Verification items for the finished model (mm, model axes). Round coordinates to 2 decimals unless told otherwise and drop trailing zeros. Write each loop counter-clockwise with the first axis right and the second up, starting at its lowest first coordinate (ties: lowest second). Pieces come first, ordered by that corner, then holes.
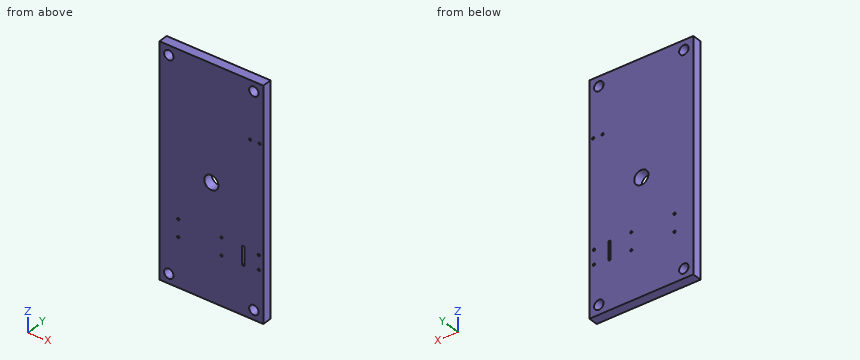
from build123d import *

# Parameters (mm, degrees)
SKETCH1_W                      = 139.7
SKETCH1_H                      = 304.8
BOSS_EXTRUDE1_DEPTH            = 12.7
SKETCH5_R                      = 6.35
CUT_EXTRUDE2_DEPTH             = 13.7
F_3_4_0_7500_DOWEL_HOLE1_D     = 19.05
F_3_4_0_7500_DOWEL_HOLE1_DEPTH = 25.4
F_3_4_0_7500_DOWEL_HOLE1_TIP   = 5.723197396
SKETCH10_R                     = 1.5
CUT_EXTRUDE3_DEPTH             = 13.7
SKETCH11_R                     = 1.5
CUT_EXTRUDE4_DEPTH             = 13.7
SKETCH12_R                     = 1.5
SKETCH12_W                     = 3.175
SKETCH12_H                     = 25
CUT_EXTRUDE6_DEPTH             = 13.7


with BuildPart() as part:
    # Sketch1 → Boss-Extrude1 (new body)
    with BuildSketch(Plane(origin=(0, 0, 0), x_dir=(1, 0, 0), z_dir=(0, 1, 0))):
        with Locations((69.85, 152.4)):
            Rectangle(SKETCH1_W, SKETCH1_H)
    extrude(amount=BOSS_EXTRUDE1_DEPTH)

    # Sketch5 → Cut-Extrude2 (cut, through all)
    with BuildSketch(Plane(origin=(0, 12.7, 0), x_dir=(1, 0, 0), z_dir=(0, 1, 0))):
        with Locations((12.7, 12.7)):
            Circle(SKETCH5_R)
        with Locations((127, 12.7)):
            Circle(SKETCH5_R)
        with Locations((127, 292.1)):
            Circle(SKETCH5_R)
        with Locations((12.7, 292.1)):
            Circle(SKETCH5_R)
    extrude(amount=-CUT_EXTRUDE2_DEPTH, mode=Mode.SUBTRACT)

    # 3/4 (0.7500) Dowel Hole1
    with Locations(Plane(origin=(69.85, 12.7, -152.4), x_dir=(0, 0, 1), z_dir=(0, 1, 0))):
        with Locations((0, 0)):
            Hole(F_3_4_0_7500_DOWEL_HOLE1_D / 2, depth=F_3_4_0_7500_DOWEL_HOLE1_DEPTH)
            with Locations((0, 0, -(F_3_4_0_7500_DOWEL_HOLE1_DEPTH + F_3_4_0_7500_DOWEL_HOLE1_TIP / 2))):  # 118° drill point
                Cone(0, F_3_4_0_7500_DOWEL_HOLE1_D / 2, F_3_4_0_7500_DOWEL_HOLE1_TIP, mode=Mode.SUBTRACT)

    # Sketch10 → Cut-Extrude3 (cut, through all)
    with BuildSketch(Plane(origin=(0, 12.7, 0), x_dir=(1, 0, 0), z_dir=(0, 1, 0))):
        with Locations((25.4, 217.0999976)):
            Circle(SKETCH10_R)
        with Locations((25.4, 240.1000024)):
            Circle(SKETCH10_R)
        with Locations((83.400011, 240.1000024)):
            Circle(SKETCH10_R)
        with Locations((83.400011, 217.0999976)):
            Circle(SKETCH10_R)
    extrude(amount=-CUT_EXTRUDE3_DEPTH, mode=Mode.SUBTRACT)

    # Sketch11 → Cut-Extrude4 (cut, through all)
    with BuildSketch(Plane(origin=(0, 12.7, 0), x_dir=(1, 0, 0), z_dir=(0, 1, 0))):
        with Locations((134.62, 76.2)):
            Circle(SKETCH11_R)
        with Locations((121.92, 76.2)):
            Circle(SKETCH11_R)
    extrude(amount=-CUT_EXTRUDE4_DEPTH, mode=Mode.SUBTRACT)

    # Sketch12 → Cut-Extrude6 (cut, through all)
    with BuildSketch(Plane(origin=(0, 12.7, 0), x_dir=(1, 0, 0), z_dir=(0, 1, 0))):
        with Locations((133.52, 219.09999995)):
            Circle(SKETCH12_R)
        with Locations((133.52, 238.10000005)):
            Circle(SKETCH12_R)
        with Locations((112.7125, 228.6)):
            Rectangle(SKETCH12_W, SKETCH12_H)
    extrude(amount=-CUT_EXTRUDE6_DEPTH, mode=Mode.SUBTRACT)


solid = part.part
Q1. Sectioned sample at D-D (y = 7.75). Give the number of separate pieces and of enclosed holes in the cut face, plus the area to 3 significant figures.
Recorded:
separate pieces: 1
enclosed holes: 14
area: 41,700 mm2
Q2. Material ranges on line 1 along Z through (x, y) = (127, 4.25); line 2 along Z through (x, y) = (25.4, 10); line 3 along X through (y, z) = (12.25, -231.5) (3 decimals), recorded low to high.
Recorded:
line 1: z = -304.8 to -298.45, -285.75 to -19.05, -6.35 to 0
line 2: z = -304.8 to -241.6, -238.6 to -218.6, -215.6 to 0
line 3: x = 0 to 111.125, 114.3 to 139.7
Q3. Sectioned sample at A-A (x = 12.7). Enter the section's corners in (y, z).
Recorded:
outline: (0, -304.8) - (12.7, -304.8) - (12.7, -298.45) - (0, -298.45) - close; (0, -285.75) - (12.7, -285.75) - (12.7, -19.05) - (0, -19.05) - close; (0, -6.35) - (12.7, -6.35) - (12.7, 0) - (0, 0) - close
Q4. Sectioned sample at B-B (z = -152.4). Enter the section's corners in (x, y) (3 decimals).
Recorded:
outline: (0, 0) - (60.325, 0) - (60.325, 12.7) - (0, 12.7) - close; (79.375, 0) - (139.7, 0) - (139.7, 12.7) - (79.375, 12.7) - close
Q5. Sectioned sample at C-C (z = -12.7). Enter the section's corners in (x, y), plus the area to 3 significant figures.
Recorded:
outline: (0, 0) - (6.35, 0) - (6.35, 12.7) - (0, 12.7) - close; (19.05, 0) - (120.65, 0) - (120.65, 12.7) - (19.05, 12.7) - close; (133.35, 0) - (139.7, 0) - (139.7, 12.7) - (133.35, 12.7) - close
area: 1,450 mm2
